The drawing under review shows one solid part. Ordinate dimensions are in mm from its lowest x, y, z. Round coordinates to 2 decimals unless told otherwise and drop trailing zeros. Write each loop counter-clockwise with the first axis right and the second up, starting at its lowest first coordinate (ties: lowest second). Pieces come first, ordered by that corner, then holes. Notation, with made-up numbers: M 80,-37 L 120,-37 A29 cw 120,-14 Z; hole C -33,10 d3. An arc over 180 degrees is marked long. Write item = value, one per line. Start each with the question number.
Item 1: Take a section at D-D, the plane x = 21.5. Give the boundary of the cut face in (y, z) (1 decimal).
Item 2: The part is to be moulded in two halves that separate along Z. For the marked faces 1, 2, 3 and 4, say which applies: +Z half, -Z half, draft (parallel to the pull), parting line (faces both ways), or undercut.
Item 3: For pin 1 Ø2 at (y, z) = (3, 16) entering from +X; pin 2 Ø0.8 at (x, y) = (30, 2) entering from +Z (1 decimal); pin 3 Ø0.6 at (y, z) = (2.5, 16.5) entering from -X; pin 4 Ø0.8 at (x, z) = (1.27, 16.51) entering from -Y, all flat-tipped, find the tip position at first contact; note any pin that passes through.
Item 4: Take a section at A-A, the plane y = 2.6. Give the boundary of the cut face in (x, z) (1 decimal), plus the area to 3 significant figures.
Item 5: To check wall thickness, follow line 1 along X through (y, z) = (0.5, 1.27) (1 decimal); line 2 along Z through (x, y) = (41.91, 0.65) (1 decimal); line 3 along Z through (x, y) = (26.5, 3.5) (1 decimal). State the ranges of each line that lie inside material, in increasing order.
Item 6: Take a section at B-B, the plane x = 1.27. Give the boundary of the cut face in (y, z) (1 decimal).
Item 7: Take a section at C-C, the plane z = 16.51. Give the boundary of the cut face in (x, y) (1 decimal).
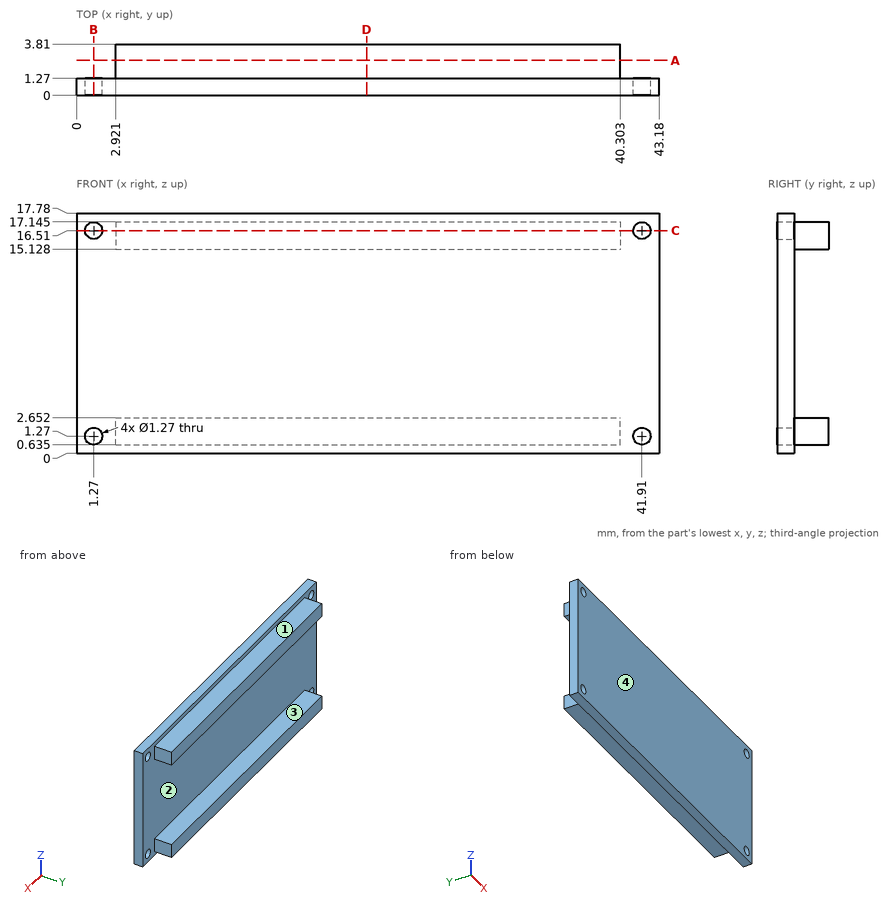
Response values:
q1.outline = M 0,0 L 1.3,0 L 1.3,0.6 L 3.8,0.6 L 3.8,2.7 L 1.3,2.7 L 1.3,15.1 L 3.8,15.1 L 3.8,17.1 L 1.3,17.1 L 1.3,17.8 L 0,17.8 Z
q2.face_1 = +Z half
q2.face_2 = undercut
q2.face_3 = undercut
q2.face_4 = draft
q3.pin_1 = 40.3
q3.pin_2 = 17.1
q3.pin_3 = 2.92
q3.pin_4 = through
q4.outline = M 2.9,0.6 L 40.3,0.6 L 40.3,2.7 L 2.9,2.7 Z; M 2.9,15.1 L 40.3,15.1 L 40.3,17.1 L 2.9,17.1 Z
q4.area = 151 mm2
q5.line_1 = 0 to 0.6, 1.9 to 41.3, 42.5 to 43.2
q5.line_2 = 0 to 0.6, 1.9 to 15.9, 17.1 to 17.8
q5.line_3 = 0.6 to 2.7, 15.1 to 17.1
q6.outline = M 0,0 L 1.3,0 L 1.3,0.6 L 0,0.6 Z; M 0,1.9 L 1.3,1.9 L 1.3,15.9 L 0,15.9 Z; M 0,17.1 L 1.3,17.1 L 1.3,17.8 L 0,17.8 Z
q7.outline = M 0,0 L 0.6,0 L 0.6,1.3 L 0,1.3 Z; M 1.9,0 L 41.3,0 L 41.3,1.3 L 40.3,1.3 L 40.3,3.8 L 2.9,3.8 L 2.9,1.3 L 1.9,1.3 Z; M 42.5,0 L 43.2,0 L 43.2,1.3 L 42.5,1.3 Z
